Build history of the part. All positions in model axes, mm. Round coordinates to 2 decimals unless told otherwise and drop trailing zeros. Order: outer loops, then holes, each group sorted by start corner. A loop starts at its lowest first (then second) coordinate and runs counter-clockwise, first axis right, second up. Notation, with made-up numbers: M 58,69 L 111,69 A30 ccw 111,91 Z; hole C 75.5,31.25 d5. An arc over 180 degrees is marked long. Use CSV: the item, a comma, the result in double quotes.
from build123d import *

# Parameters (mm, degrees)
F0_R     = 4
F1_DEPTH = 10
F2_D     = 4.4
F2_DEPTH = 10
F2_TIP   = 1.3218933619


with BuildPart() as f1:
    # F0 (on Front) → F1 (new body)
    with BuildSketch(Plane.XZ):
        with BuildLine():
            Line((-13, -7.5), (13, -7.5))
            ThreePointArc((13, -7.5), (20.5, 0), (13, 7.5))
            Line((13, 7.5), (-13, 7.5))
            ThreePointArc((-13, 7.5), (-20.5, 0), (-13, -7.5))
        make_face()
        Circle(F0_R, mode=Mode.SUBTRACT)
    extrude(amount=-F1_DEPTH)

    # F2
    with Locations(Plane.XZ):
        with Locations((-13, 0), (13, 0)):
            Hole(F2_D / 2, depth=F2_DEPTH)
            with Locations((0, 0, -(F2_DEPTH + F2_TIP / 2))):  # 118° drill point
                Cone(0, F2_D / 2, F2_TIP, mode=Mode.SUBTRACT)


solid = f1.part
(1) Cut at C-C, the plane x = 2. Give the cut face in (y, z), and give its area (3 significant figures).
Answer block:
outline,"M 0,-7.5 L 10,-7.5 L 10,-3.46 L 0,-3.46 Z; M 0,3.46 L 10,3.46 L 10,7.5 L 0,7.5 Z"
area,"80.7 mm²"
(2) Drop flat-ended pins along their axis: pin 1 (1.5 mm diameter, centred on y = 4, z = -1, fed in from +X); pin 2 (2 mm diameter, centred on x = -16, y = 4, fed in from -Z). Give the stop position or say it passes through.
Answer block:
pin 1,"stops at x = 20.5"
pin 2,"stops at z = -7.23"
(3) Two-plate mould, pull along Z, no slides. Class faces 1 (the face through (-0.867, 4.93, -3.905)), 2 (the face through (4.3, 0, 0.1)), 3 (the face through (10.968, 5.07, -0.843)), 4 (the face through (20.5, 4.93, -0.16)): released by +Z, released by -Z, zero draft, split by the parting line, or undercut.
Answer block:
face 1,"undercut"
face 2,"zero draft"
face 3,"undercut"
face 4,"split by the parting line"
(4) Wall check: line 1 (Z direction, x = -13, y = 6); line 2 (Z direction, x = 0, y = 6.25); line 3 (X direction, y = 3.5, z = -0.25). Give the ranges that are in metal, low to high. Write a range as from..to.
Answer block:
line 1,"z = -7.5..-2.2, 2.2..7.5"
line 2,"z = -7.5..-4, 4..7.5"
line 3,"x = -20.5..-15.19, -10.81..-3.99, 3.99..10.81, 15.19..20.5"
(5) Cut at A-A, the plane x = -12. Give the cut face in (y, z), and give its area (3 significant figures).
Answer block:
outline,"M 0,-7.5 L 10,-7.5 L 10,-1.96 L 0,-1.96 Z; M 0,1.96 L 10,1.96 L 10,7.5 L 0,7.5 Z"
area,"111 mm²"
(6) Cut at B-B, the plane y = 5.75. Give the cut face in (x, z), and give its area (3 significant figures).
Answer block:
outline,"M -13,-7.5 L 13,-7.5 A7.5 ccw 13,7.5 L -13,7.5 A7.5 ccw Z; hole C -13,0 d4.4; hole C 0,0 d8; hole C 13,0 d4.4"
area,"486 mm²"
